Source: CAD feature listing. Evaluate the final solid. Frame: model axes, mm. Face numbers are marked on the shaded views. A direction names the side the tool comes from. Round coordinates to 2 decimals unless told otherwise and drop trailing zeros. Order: outer loops, then holes, each group sorted by start corner. A loop starts at its lowest first (then second) coordinate and runs counter-clockwise, first axis right, second up. Notation, with made-up numbers: (41.25, -28.75) - (83.25, -28.75) arc R13 cw to (83.25, -20.75) - close; hole circle Ø11 at (-19.75, 2.5). An arc over 180 degrees is marked (long way). Return JSON: item names as keys, results as strings. Group by question number.
1) Section D-D, the plane z = -10. Return loops of the section in (x, y).
2) Contact query for flat-ended pins moving along their axis: P1, Ø8, axis at x = 8, z = -7, coming from the -Y side; P2, Ø4, axis at x = 22, y = 22, coming from the +Z side; P3, Ø1.8, axis at x = 26.5, y = 22, coming from the -Z side. Output: stop coordinate, or through.
3) Section A-A, the plane x = 0. Return loops of the section in (y, z).
4) Ray query, line 1 (X direction, y = 14.75, z = 4); line 2 (Y direction, x = 0, z = 13). Return the intervals inside material, ascending. Write a range as from..to.
5) Mould query, pull axis Z, two halves, no side actions, for the marked faces 4, 5 and 6. Classes: pulls with the +Z half, pulls with the -Z half, needs draft (parallel to the pull), parting line crosses it, or undercut.
6) Access query for the marked faces 1, 2 and 3. Directions: +Z, -Z, +X, -X, +Y, -Y. A direction counts if a zero-diameter tool reaches every point of the face in a straight line with its end or side. Return the directions, or none.
7) Section C-C, the plane x = -7.5. Return loops of the section in (y, z).
8) Section B-B, the plane y = 15.5. Return loops of the section in (x, z), plus the area to 3 significant figures.
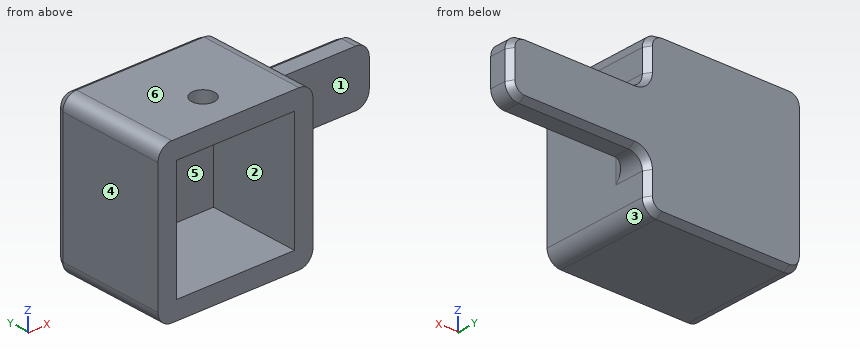
```python
from build123d import *
from OCP.BRepFilletAPI import BRepFilletAPI_MakeChamfer

# Parameters (mm, degrees)
SKETCH1_W           = 33.8
SKETCH1_H           = 33.8
SKETCH1_W_2         = 25.8
SKETCH1_H_2         = 25.8
BOSS_EXTRUDE1_DEPTH = 20
SKETCH2_W           = 30
SKETCH2_H           = 12
SKETCH2_W_2         = 25.8
SKETCH2_H_2         = 25.8
BOSS_EXTRUDE2_DEPTH = 5
CUT_EXTRUDE1_REACH  = 64.985
SKETCH3_R           = 2.5
FILLET1_R           = 3
CHAMFER1_SIZE       = 1.5
CHAMFER1_SIZE2      = 0.866025404


with BuildPart() as part:
    # Sketch1 → Boss-Extrude1 (new body)
    with BuildSketch(Plane(origin=(0, 0, 0), x_dir=(1, 0, 0), z_dir=(0, 1, 0))):
        Rectangle(SKETCH1_W, SKETCH1_H)
        Rectangle(SKETCH1_W_2, SKETCH1_H_2, mode=Mode.SUBTRACT)
    extrude(amount=BOSS_EXTRUDE1_DEPTH)

    # Sketch2 → Boss-Extrude2 (add)
    # profile 1 of 3: a face of its own
    with BuildSketch(Plane(origin=(0, 20, 0), x_dir=(1, 0, 0), z_dir=(0, 1, 0))):
        with Locations((31.9, 0)):
            Rectangle(SKETCH2_W, SKETCH2_H)
    # profile 2 of 3: a face of its own
    with BuildSketch(Plane(origin=(0, 20, 0), x_dir=(1, 0, 0), z_dir=(0, 1, 0))):
        Polygon((16.9, 16.9), (-16.9, 16.9), (-16.9, -16.9), (16.9, -16.9), (16.9, -6), (16.9, 6), align=None)
        Rectangle(SKETCH2_W_2, SKETCH2_H_2, mode=Mode.SUBTRACT)
    # profile 3 of 3: a face of its own
    with BuildSketch(Plane(origin=(0, 20, 0), x_dir=(1, 0, 0), z_dir=(0, 1, 0))):
        Rectangle(SKETCH2_W_2, SKETCH2_H_2)
    extrude(amount=BOSS_EXTRUDE2_DEPTH)

    # Sketch3 → Cut-Extrude1 (cut, up to next)
    with BuildSketch(Plane.XY.offset(16.9), mode=Mode.PRIVATE) as cut_extrude1_sk1:
        with Locations((0, 8)):
            Circle(SKETCH3_R)
    cut_extrude1_tool1 = extrude(cut_extrude1_sk1.sketch, amount=-CUT_EXTRUDE1_REACH, mode=Mode.PRIVATE) & part.part
    add(cut_extrude1_tool1.solids().sort_by_distance((0, 8, 16.9))[0], mode=Mode.SUBTRACT)

    # Fillet1
    fillet1_edges = [part.edges().sort_by_distance(p)[0] for p in [
        (16.9, 20, 0),
        (16.9, 22.5, 6),
        (46.9, 22.5, 6),
        (46.9, 22.5, -6),
        (16.9, 22.5, -6),
        (-16.9, 12.5, 16.9),
        (-16.9, 12.5, -16.9),
        (16.9, 12.5, -16.9),
        (16.9, 12.5, 16.9),
    ]]
    fillet(fillet1_edges, radius=FILLET1_R)

    # Chamfer1: one chamfer whose edges measure the first distance from different faces: ONE call of the kernel's chamfer builder (chamfer() names one face for all edges)
    chamfer1_edges_1 = [part.edges().sort_by_distance(p)[0] for p in [
        (16.9, 25, -11.45),
        (16.9, 25, 11.45),
    ]]
    chamfer1_side_1 = [part.faces().sort_by_distance(p)[0] for p in [
        (16.9, 10.278584392, 0),
    ]]
    chamfer1_edges_2 = [part.edges().sort_by_distance(p)[0] for p in [
        (0, 25, 16.9),
    ]]
    chamfer1_side_2 = [part.faces().sort_by_distance(p)[0] for p in [
        (0, 12.63082894, 16.9),
    ]]
    chamfer1_edges_3 = [part.edges().sort_by_distance(p)[0] for p in [
        (31.9, 25, 6),
    ]]
    chamfer1_side_3 = [part.faces().sort_by_distance(p)[0] for p in [
        (31.9, 22.5, 6),
    ]]
    chamfer1_edges_4 = [part.edges().sort_by_distance(p)[0] for p in [
        (46.9, 25, 0),
    ]]
    chamfer1_side_4 = [part.faces().sort_by_distance(p)[0] for p in [
        (46.9, 22.5, 0),
    ]]
    chamfer1_edges_5 = [part.edges().sort_by_distance(p)[0] for p in [
        (31.9, 25, -6),
    ]]
    chamfer1_side_5 = [part.faces().sort_by_distance(p)[0] for p in [
        (31.9, 22.5, -6),
    ]]
    chamfer1_edges_6 = [part.edges().sort_by_distance(p)[0] for p in [
        (0, 25, -16.9),
    ]]
    chamfer1_side_6 = [part.faces().sort_by_distance(p)[0] for p in [
        (0, 12.5, -16.9),
    ]]
    chamfer1_edges_7 = [part.edges().sort_by_distance(p)[0] for p in [
        (-16.9, 25, 0),
    ]]
    chamfer1_side_7 = [part.faces().sort_by_distance(p)[0] for p in [
        (-16.9, 12.5, 0),
    ]]
    chamfer1_edges_8 = [part.edges().sort_by_distance(p)[0] for p in [
        (46.021320344, 25, 5.121320344),
    ]]
    chamfer1_side_8 = [part.faces().sort_by_distance(p)[0] for p in [
        (46.021320344, 22.5, 5.121320344),
    ]]
    chamfer1_edges_9 = [part.edges().sort_by_distance(p)[0] for p in [
        (46.021320344, 25, -5.121320344),
    ]]
    chamfer1_side_9 = [part.faces().sort_by_distance(p)[0] for p in [
        (46.021320344, 22.5, -5.121320344),
    ]]
    chamfer1_edges_10 = [part.edges().sort_by_distance(p)[0] for p in [
        (16.021320344, 25, -16.021320344),
    ]]
    chamfer1_side_10 = [part.faces().sort_by_distance(p)[0] for p in [
        (16.021320344, 12.5, -16.021320344),
    ]]
    chamfer1_edges_11 = [part.edges().sort_by_distance(p)[0] for p in [
        (-16.021320344, 25, -16.021320344),
    ]]
    chamfer1_side_11 = [part.faces().sort_by_distance(p)[0] for p in [
        (-16.021320344, 12.5, -16.021320344),
    ]]
    chamfer1_edges_12 = [part.edges().sort_by_distance(p)[0] for p in [
        (-16.021320344, 25, 16.021320344),
    ]]
    chamfer1_side_12 = [part.faces().sort_by_distance(p)[0] for p in [
        (-16.021320344, 12.5, 16.021320344),
    ]]
    chamfer1_edges_13 = [part.edges().sort_by_distance(p)[0] for p in [
        (16.021320344, 25, 16.021320344),
    ]]
    chamfer1_side_13 = [part.faces().sort_by_distance(p)[0] for p in [
        (16.021320344, 12.5, 16.021320344),
    ]]
    chamfer1_edges_14 = [part.edges().sort_by_distance(p)[0] for p in [
        (17.778679656, 25, -6.878679656),
    ]]
    chamfer1_side_14 = [part.faces().sort_by_distance(p)[0] for p in [
        (17.778679656, 21, -6.878679656),
    ]]
    chamfer1_edges_15 = [part.edges().sort_by_distance(p)[0] for p in [
        (17.778679656, 25, 6.878679656),
    ]]
    chamfer1_side_15 = [part.faces().sort_by_distance(p)[0] for p in [
        (17.778679656, 21, 6.878679656),
    ]]
    chamfer1 = BRepFilletAPI_MakeChamfer(part.part.solid().wrapped)
    for e in chamfer1_edges_1:
        chamfer1.Add(CHAMFER1_SIZE, CHAMFER1_SIZE2, e.wrapped, chamfer1_side_1[0].wrapped)  # the first distance lies on this face
    for e in chamfer1_edges_2:
        chamfer1.Add(CHAMFER1_SIZE, CHAMFER1_SIZE2, e.wrapped, chamfer1_side_2[0].wrapped)  # the first distance lies on this face
    for e in chamfer1_edges_3:
        chamfer1.Add(CHAMFER1_SIZE, CHAMFER1_SIZE2, e.wrapped, chamfer1_side_3[0].wrapped)  # the first distance lies on this face
    for e in chamfer1_edges_4:
        chamfer1.Add(CHAMFER1_SIZE, CHAMFER1_SIZE2, e.wrapped, chamfer1_side_4[0].wrapped)  # the first distance lies on this face
    for e in chamfer1_edges_5:
        chamfer1.Add(CHAMFER1_SIZE, CHAMFER1_SIZE2, e.wrapped, chamfer1_side_5[0].wrapped)  # the first distance lies on this face
    for e in chamfer1_edges_6:
        chamfer1.Add(CHAMFER1_SIZE, CHAMFER1_SIZE2, e.wrapped, chamfer1_side_6[0].wrapped)  # the first distance lies on this face
    for e in chamfer1_edges_7:
        chamfer1.Add(CHAMFER1_SIZE, CHAMFER1_SIZE2, e.wrapped, chamfer1_side_7[0].wrapped)  # the first distance lies on this face
    for e in chamfer1_edges_8:
        chamfer1.Add(CHAMFER1_SIZE, CHAMFER1_SIZE2, e.wrapped, chamfer1_side_8[0].wrapped)  # the first distance lies on this face
    for e in chamfer1_edges_9:
        chamfer1.Add(CHAMFER1_SIZE, CHAMFER1_SIZE2, e.wrapped, chamfer1_side_9[0].wrapped)  # the first distance lies on this face
    for e in chamfer1_edges_10:
        chamfer1.Add(CHAMFER1_SIZE, CHAMFER1_SIZE2, e.wrapped, chamfer1_side_10[0].wrapped)  # the first distance lies on this face
    for e in chamfer1_edges_11:
        chamfer1.Add(CHAMFER1_SIZE, CHAMFER1_SIZE2, e.wrapped, chamfer1_side_11[0].wrapped)  # the first distance lies on this face
    for e in chamfer1_edges_12:
        chamfer1.Add(CHAMFER1_SIZE, CHAMFER1_SIZE2, e.wrapped, chamfer1_side_12[0].wrapped)  # the first distance lies on this face
    for e in chamfer1_edges_13:
        chamfer1.Add(CHAMFER1_SIZE, CHAMFER1_SIZE2, e.wrapped, chamfer1_side_13[0].wrapped)  # the first distance lies on this face
    for e in chamfer1_edges_14:
        chamfer1.Add(CHAMFER1_SIZE, CHAMFER1_SIZE2, e.wrapped, chamfer1_side_14[0].wrapped)  # the first distance lies on this face
    for e in chamfer1_edges_15:
        chamfer1.Add(CHAMFER1_SIZE, CHAMFER1_SIZE2, e.wrapped, chamfer1_side_15[0].wrapped)  # the first distance lies on this face
    add(Compound.cast(chamfer1.Shape()), mode=Mode.REPLACE)


solid = part.part
```
Geometry check:
{
 "1": {"outline": "(-16.9, 0) - (-12.9, 0) - (-12.9, 20) - (12.9, 20) - (12.9, 0) - (16.9, 0) - (16.9, 23.5) - (16.03, 25) - (-16.03, 25) - (-16.9, 23.5) - close"},
 "2": {"P1": "y = 20", "P2": "z = 6", "P3": "z = -6"},
 "3": {"outline": "(0, -16.9) - (23.5, -16.9) - (25, -16.03) - (25, 16.03) - (23.5, 16.9) - (10.5, 16.9) - (10.5, 12.9) - (20, 12.9) - (20, -12.9) - (0, -12.9) - close; (0, 12.9) - (5.5, 12.9) - (5.5, 16.9) - (0, 16.9) - close"},
 "4": {"line 1": "-16.9..-12.9, 12.9..16.9", "line 2": "0..5.5, 10.5..25"},
 "5": {"face 4": "needs draft", "face 5": "undercut", "face 6": "pulls with the +Z half"},
 "6": {"face 1": "+Z, -Z, +X, -Y", "face 2": "-Y", "face 3": "-Z, +X, +Y, -Y"},
 "7": {"outline": "(0, -16.9) - (23.5, -16.9) - (25, -16.03) - (25, 16.03) - (23.5, 16.9) - (0, 16.9) - (0, 12.9) - (20, 12.9) - (20, -12.9) - (0, -12.9) - close"},
 "8": {"outline": "(-16.9, -13.9) arc R3 ccw to (-13.9, -16.9) - (13.9, -16.9) arc R3 ccw to (16.9, -13.9) - (16.9, 13.9) arc R3 ccw to (13.9, 16.9) - (-13.9, 16.9) arc R3 ccw to (-16.9, 13.9) - close; hole (-12.9, -12.9) - (12.9, -12.9) - (12.9, 12.9) - (-12.9, 12.9) - close", "area": "469 mm2"}
}
